For this review, take the finished solid that the model builds, in its own axes (mm). Round coordinates to 2 decimals unless told otherwise and drop trailing zeros. Order: outer loops, then holes, each group sorted by start corner. A loop starts at its lowest first (then second) coordinate and runs counter-clockwise, first axis right, second up. Notation, with made-up numbers: M -29,16.25 L -18,16.25 A32 cw -18,52.25 Z; hole C 26.25,30 d1. An arc over 180 degrees is marked long. Use a Markdown table: item, result.
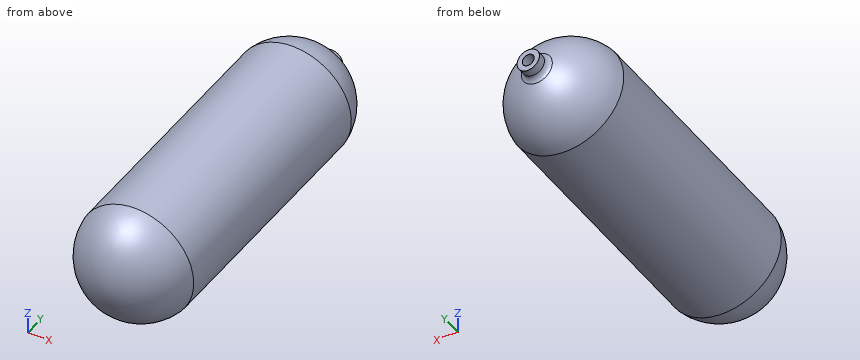
from build123d import *

# Parameters (mm, degrees)
Y_KSEKLIK_EKSTR_ZYON1_DEPTH      = 195
Y_KSEKLIK_EKSTR_ZYON1_DEPTH_BACK = 195
IZIM2_R                          = 87.5
IZIM2_R_2                        = 79.5
RADYUS1_R                        = 9


with BuildPart() as part:
    # izim2 → Y_kseklik-Ekstr_zyon1 (new, two sides: drawn at the far end of the back side and taken through both)
    with BuildSketch(Plane(origin=(0, 0, 0), x_dir=(1, 0, 0), z_dir=(0, 1, 0)).offset(-Y_KSEKLIK_EKSTR_ZYON1_DEPTH_BACK)):
        with Locations(Location((0, 0, 0), (0, 0, 270))):
            Circle(IZIM2_R)
        with Locations(Location((0, 0, 0), (0, 0, 270))):
            Circle(IZIM2_R_2, mode=Mode.SUBTRACT)
    extrude(amount=Y_KSEKLIK_EKSTR_ZYON1_DEPTH + Y_KSEKLIK_EKSTR_ZYON1_DEPTH_BACK)

    # izim3 → D_nd_r1 (revolve)
    with BuildSketch(Plane(origin=(0, 0, 0), x_dir=(0, 0, -1), z_dir=(1, 0, 0))):
        with BuildLine():
            ThreePointArc((-9.086559343, 262.571806636), (-55.708005592, 240.680658931), (-79.5, 195))
            Line((-79.5, 195), (-87.5, 195))
            ThreePointArc((-87.5, 195), (-64.125045155, 243.434926699), (-17, 269.349416033))
            Line((-17, 269.349416033), (-17, 289))
            Line((-17, 289), (-9, 289))
            Line((-9, 289), (-9.086559343, 262.571806636))
        make_face()
    revolve(axis=Axis((0, 271, 0), (0, -1, 0)))

    # izim4 → D_nd_r2 (revolve)
    with BuildSketch(Plane(origin=(0, 0, 0), x_dir=(0, 0, -1), z_dir=(1, 0, 0)), mode=Mode.PRIVATE) as d_nd_r2_sk:
        with BuildLine():
            Line((87.5, -195), (79.5, -195))
            ThreePointArc((79.5, -195), (52.335527042, -243.73853538), (0, -263.086559343))
            Line((0, -263.086559343), (0, -271))
            ThreePointArc((0, -271), (57.94879205, -249.347293478), (87.5, -195))
        make_face()
    revolve(d_nd_r2_sk.sketch.rotate(Axis((0, 271, 0), (0, -1, 0)), 180), axis=Axis((0, 271, 0), (0, -1, 0)))

    # Radyus1
    radyus1_edges = [part.edges().sort_by_distance(p)[0] for p in [
        (0, 269.349416033, -17),
    ]]
    fillet(radyus1_edges, radius=RADYUS1_R)


solid = part.part
Q1. Add section C-C (y = 89.5). Write out the cut boundary in (x, z), then the cut area to 3 significant figures.
Determined:
| item | result |
|---|---|
| outline | C 0,0 d175; hole C 0,0 d159 |
| area | 4,200 mm^2 |
Q2. Add section A-A (z = -74). Write out the cut boundary in (x, y), then the cut area to 3 significant figures.
Determined:
| item | result |
|---|---|
| outline | M -46.69,-195 A48.3 ccw 46.69,-195 L 46.69,195 A48.3 ccw -46.69,195 Z; hole M -29.06,-195 A31.58 ccw 29.06,-195 L 29.06,195 A31.58 ccw -29.06,195 Z |
| area | 17,100 mm^2 |
Q3. Wall thickness on line 1 along X through (y, z) = (38, 0); line 2 along X through (y, z) = (194.5, 4); line 3 along Y through (x, z) = (-27.5, 4.5): over which ranges is each line inside the solid? List them lowest first. Write a range as [from, to].
Determined:
| item | result |
|---|---|
| line 1 | x = [-87.5, -79.5], [79.5, 87.5] |
| line 2 | x = [-87.41, -79.4], [79.4, 87.41] |
| line 3 | y = [-266.49, -258.11], [258.11, 266.49] |
Q4. Clearance check with flat-ended pins moving along their axes: pin 1 (12 mm diameter, centred on y = 218.5, z = 42.5, fed in from +X); pin 2 (5 mm diameter, centred on y = 176, z = 24, fed in from -X); pin 3 (8 mm diameter, centred on x = -26, z = -31, fed in from +Y). State where each tip first meets the part, or that it passes through.
Determined:
| item | result |
|---|---|
| pin 1 | stops at x = 73.13 |
| pin 2 | stops at x = -84.82 |
| pin 3 | stops at y = 263.13 |
Q5. Add section B-B (x = 61.5). Write out the cut boundary in (y, z), then the cut area to 3 significant figures.
Determined:
| item | result |
|---|---|
| outline | M -195,-62.24 L 195,-62.24 A63.46 ccw 195,62.24 L -195,62.24 A63.46 ccw Z; hole M -195,-50.38 L 195,-50.38 A51.88 ccw 195,50.38 L -195,50.38 A51.88 ccw Z |
| area | 12,900 mm^2 |
